from build123d import *

# Parameters (mm, degrees)
F0_W     = 63.8
F0_H     = 31.7
F1_DEPTH = 9.6
F2_R     = 4.7
F2_R_2   = 3.4
F3_DEPTH = 4.6


with BuildPart() as f1:
    # F0 (on Top) → F1 (new body)
    with BuildSketch(Plane.XY):
        Rectangle(F0_W, F0_H)
    extrude(amount=F1_DEPTH)

    # F2 (on face) → F3 (join)
    with BuildSketch(Plane.XY.offset(9.6)):
        with Locations((7.95, 7.95)):
            Circle(F2_R)
        with Locations((7.95, 7.95)):
            Circle(F2_R_2, mode=Mode.SUBTRACT)
        with Locations((-7.95, 7.95)):
            Circle(F2_R)
        with Locations((-7.95, 7.95)):
            Circle(F2_R_2, mode=Mode.SUBTRACT)
        with Locations((-23.85, 7.95)):
            Circle(F2_R)
        with Locations((-23.85, 7.95)):
            Circle(F2_R_2, mode=Mode.SUBTRACT)
        with Locations((23.85, 7.95)):
            Circle(F2_R)
        with Locations((23.85, 7.95)):
            Circle(F2_R_2, mode=Mode.SUBTRACT)
        with Locations((7.95, -7.95)):
            Circle(F2_R)
        with Locations((7.95, -7.95)):
            Circle(F2_R_2, mode=Mode.SUBTRACT)
        with Locations((-23.85, -7.95)):
            Circle(F2_R)
        with Locations((-23.85, -7.95)):
            Circle(F2_R_2, mode=Mode.SUBTRACT)
        with Locations((23.85, -7.95)):
            Circle(F2_R)
        with Locations((23.85, -7.95)):
            Circle(F2_R_2, mode=Mode.SUBTRACT)
        with Locations((-7.95, -7.95)):
            Circle(F2_R)
        with Locations((-7.95, -7.95)):
            Circle(F2_R_2, mode=Mode.SUBTRACT)
    extrude(amount=F3_DEPTH)


solid = f1.part
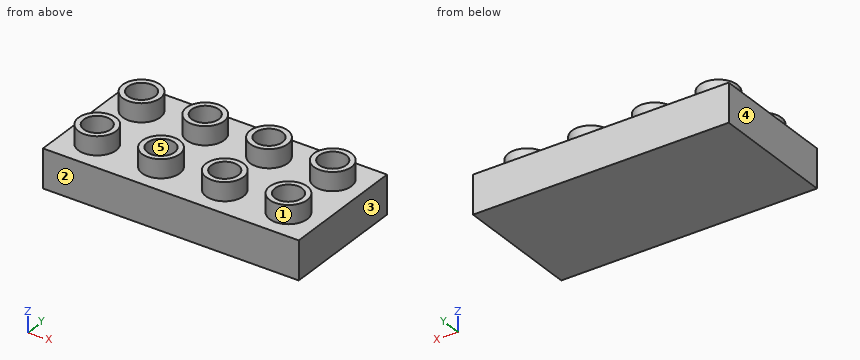
Source: CAD feature listing. Evaluate the final solid. Frame: model axes, mm. Face numbers are marked on the shaded views. A direction names the side the tool comes from. Coordinates: 2 decimals unless noted, no trailing zeros. Write each loop counter-clockwise with the first axis right and the second up, starting at its lowest first coordinate (ties: lowest second). Pieces come first, ordered by that corner, then holes. Notation, with made-up numbers: M 20,-15.75 L 32,-15.75 A17 ccw 32,14.25 Z; hole C 42,-31.5 d9. An arc over 180 degrees is marked long. Use a Markdown table: item, result.
1) Section D-D, the plane x = 16. Output: boundary loops of the cut face in (y, z), then the cut area to 3 significant figures.
Conclusion:
| item | result |
|---|---|
| outline | M -15.85,0 L 15.85,0 L 15.85,9.6 L -15.85,9.6 Z |
| area | 304 mm^2 |
2) Section C-C, the plane y = -14. Output: boundary loops of the cut face in (x, z).
Conclusion:
| item | result |
|---|---|
| outline | M -31.9,0 L 31.9,0 L 31.9,9.6 L -31.9,9.6 Z |
3) Section A-A, the plane z = 10.5. Give the number of separate pieces and of enclosed holes in the cut face, then the cut area to 3 significant figures.
Conclusion:
| item | result |
|---|---|
| separate pieces | 8 |
| enclosed holes | 8 |
| area | 265 mm^2 |
4) Reachability of the marked faces 4 and 5 from +Z, -Z, +X, -X, +Y, -Y: full face, straight path, thin tool, end or side. Return the list, or none.
Conclusion:
| item | result |
|---|---|
| face 4 | +Z, -Z, -X, +Y, -Y |
| face 5 | +Z |
5) Section B-B, the plane x = -23.85. Output: boundary loops of the cut face in (y, z), then the cut area to 3 significant figures.
Conclusion:
| item | result |
|---|---|
| outline | M -15.85,0 L 15.85,0 L 15.85,9.6 L 12.65,9.6 L 12.65,14.2 L 11.35,14.2 L 11.35,9.6 L 4.55,9.6 L 4.55,14.2 L 3.25,14.2 L 3.25,9.6 L -3.25,9.6 L -3.25,14.2 L -4.55,14.2 L -4.55,9.6 L -11.35,9.6 L -11.35,14.2 L -12.65,14.2 L -12.65,9.6 L -15.85,9.6 Z |
| area | 328 mm^2 |
6) First-contact query: pin 1 Ø4 at (x, z) = (-6, 11) entering from +Y; pin 2 Ø4 at (x, y) = (-7.95, 7.95) entering from +Z. Flat tips, straight axial feed; report the tip coordinate or a pass-through.
Conclusion:
| item | result |
|---|---|
| pin 1 | stops at y = 15.85 |
| pin 2 | stops at z = 9.6 |
7) Mould query, pull axis Y, two halves, no side actions, for the marked faces 1, 2 and 3. Classes: pulls with the +Y half, pulls with the -Y half, needs draft (parallel to the pull), parting line crosses it, or undercut.
Conclusion:
| item | result |
|---|---|
| face 1 | undercut |
| face 2 | pulls with the -Y half |
| face 3 | needs draft |
8) Ray query, L1, parallel to Y at x = -7.95, z = 10.8; L2, parallel to Z at x = 15, y = 2.5; L3, parallel to X at y = 4, z = 11. Return the intervals inside material, ascending.
Conclusion:
| item | result |
|---|---|
| L1 | y = -12.65 to -11.35, -4.55 to -3.25, 3.25 to 4.55, 11.35 to 12.65 |
| L2 | z = 0 to 9.6 |
| L3 | x = -26.4 to -21.3, -10.5 to -5.4, 5.4 to 10.5, 21.3 to 26.4 |
